Input: part model. Units: mm. Frame: model coordinates. Face numbers are marked on the shaded views. A direction names the side the tool comes from. Coordinates: 2 decimals unless noted, no trailing zeros. Order: outer loops, then holes, each group sorted by start corner. A loop starts at its lowest first (then second) coordinate and runs counter-clockwise, first axis right, second up. Notation, with made-up numbers: (82, -21.5) -> (115, -21.5) arc R19 ccw to (115, -9.5) -> close; hole circle Ø1 at (-15.5, -25). An arc over 180 degrees is marked (long way). One line per question, with ' | ' between items.
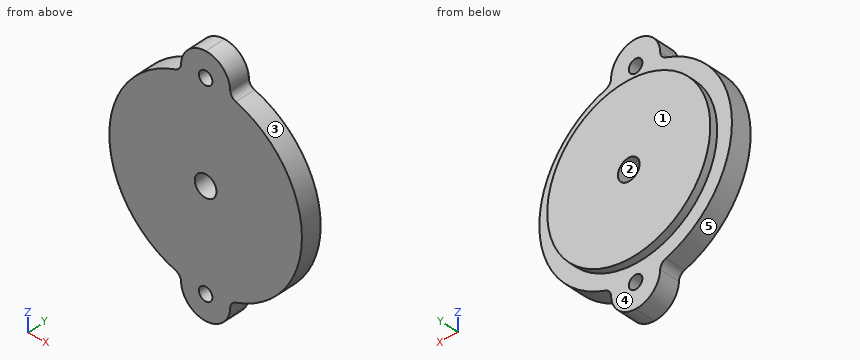
```python
from build123d import *

# Parameters (mm, degrees)
SKETCH1_W           = 60
SKETCH1_H           = 60
SKETCH1_R           = 1.65
BOSS_EXTRUDE1_DEPTH = 5
SKETCH2_R           = 19.9
BOSS_EXTRUDE2_DEPTH = 1.83
SKETCH3_OUTSIDE_W   = 79.026
SKETCH3_OUTSIDE_H   = 79.026
CUT_EXTRUDE1_DEPTH  = 43.720018727
SKETCH4_R           = 2.65
CUT_EXTRUDE2_DEPTH  = 39.715615713
FILLET1_R           = 2


with BuildPart() as part:
    # Sketch1 → Boss-Extrude1 (new body)
    with BuildSketch(Plane(origin=(0, 0, 0), x_dir=(1, 0, 0), z_dir=(0, 1, 0))):
        Rectangle(SKETCH1_W, SKETCH1_H)
        with Locations(Location((0, 24, 0), (0, 0, 270))):
            Circle(SKETCH1_R, mode=Mode.SUBTRACT)
        with Locations(Location((0, -24, 0), (0, 0, 270))):
            Circle(SKETCH1_R, mode=Mode.SUBTRACT)
    extrude(amount=BOSS_EXTRUDE1_DEPTH)

    # Sketch2 → Boss-Extrude2 (add)
    with BuildSketch(Plane(origin=(0, 5, 0), x_dir=(1, 0, 0), z_dir=(0, 1, 0))):
        with Locations(Location((0, 0, 0), (0, 0, 270))):
            Circle(SKETCH2_R)
    extrude(amount=BOSS_EXTRUDE2_DEPTH)

    # Sketch3 outside → Cut-Extrude1 (cut, through all)
    with BuildSketch(Plane(origin=(0, 5, 0), x_dir=(1, 0, 0), z_dir=(0, 1, 0))):
        Rectangle(SKETCH3_OUTSIDE_W, SKETCH3_OUTSIDE_H)
        with BuildLine():
            ThreePointArc((5.869454294, -22.755208333), (23.5, 0), (5.869454294, 22.755208333))
            ThreePointArc((5.869454294, 22.755208333), (4.66201405, 27.776986232), (0, 30))
            ThreePointArc((0, 30), (-4.66201405, 27.776986232), (-5.869454294, 22.755208333))
            ThreePointArc((-5.869454294, 22.755208333), (-23.5, 0), (-5.869454294, -22.755208333))
            ThreePointArc((-5.869454294, -22.755208333), (-4.66201405, -27.776986232), (0, -30))
            ThreePointArc((0, -30), (4.66201405, -27.776986232), (5.869454294, -22.755208333))
        make_face(mode=Mode.SUBTRACT)
    extrude(amount=-CUT_EXTRUDE1_DEPTH, mode=Mode.SUBTRACT)

    # Sketch4 → Cut-Extrude2 (cut, through all)
    with BuildSketch(Plane.XZ):
        with Locations(Location((0, 0, 0), (0, 0, 270))):
            Circle(SKETCH4_R)
    extrude(amount=-CUT_EXTRUDE2_DEPTH, mode=Mode.SUBTRACT)

    # Fillet1
    fillet1_edges = [part.edges().sort_by_distance(p)[0] for p in [
        (5.869454294, 2.5, -22.755208333),
        (-5.869454294, 2.5, 22.755208333),
        (5.869454294, 2.5, 22.755208333),
        (-5.869454294, 2.5, -22.755208333),
    ]]
    fillet(fillet1_edges, radius=FILLET1_R)


solid = part.part
```
1. Cut plane C-C, the plane z = 6.5. Return loops of the section in (x, y).
Recorded:
outline: (-22.58, 0) -> (22.58, 0) -> (22.58, 5) -> (18.81, 5) -> (18.81, 6.83) -> (-18.81, 6.83) -> (-18.81, 5) -> (-22.58, 5) -> close
2. Ray query, line 1 (X direction, y = 1.55, z = 24); line 2 (Z direction, x = -1, y = 0.75); line 3 (Y direction, x = -15, z = 16.5). Return the intervals inside material, ascending. Write a range as [from, to].
Recorded:
line 1: x = [-6.01, -1.65], [1.65, 6.01] | line 2: z = [-29.92, -25.31], [-22.69, -2.45], [2.45, 22.69], [25.31, 29.92] | line 3: y = [0, 5]
3. Cut plane B-B, the plane x = 17. Return loops of the section in (y, z).
Recorded:
outline: (0, -16.22) -> (5, -16.22) -> (5, -10.34) -> (6.83, -10.34) -> (6.83, 10.34) -> (5, 10.34) -> (5, 16.22) -> (0, 16.22) -> close
4. Mould query, pull axis Z, two halves, no side actions, for the marked faces 1, 2 and 3. Classes: released by +Z, released by -Z, zero draft, split by the parting line, or undercut.
Recorded:
face 1: zero draft | face 2: undercut | face 3: split by the parting line
5. Cut plane A-A, the plane z = 0. Return loops of the section in (x, y).
Recorded:
outline: (-23.5, 0) -> (-2.65, 0) -> (-2.65, 6.83) -> (-19.9, 6.83) -> (-19.9, 5) -> (-23.5, 5) -> close; (2.65, 0) -> (23.5, 0) -> (23.5, 5) -> (19.9, 5) -> (19.9, 6.83) -> (2.65, 6.83) -> close
6. Pin query (flat end, axial travel): pin 1 Ø4 at (y, z) = (1.5, 14.5) entering from -X; pin 2 Ø2 at (x, z) = (0.5, -22.5) entering from +Y. Return the tip coordinate at first contact, or that it passes through.
Recorded:
pin 1: stops at x = -19.9 | pin 2: stops at y = 5
7. Cut plane D-D, the plane y = 3. State how many separate pieces and enclosed holes the cut face has, and give its area (3 significant figures).
Recorded:
separate pieces: 1 | enclosed holes: 3 | area: 1,830 mm^2
8. Access query for the marked faces 4 and 5. Directions: +Z, -Z, +X, -X, +Y, -Y. A direction counts if a zero-diameter tool reaches every point of the face in a straight line with its end or side. Return the directions, or none.
Recorded:
face 4: +Y | face 5: -X, +Y, -Y
